Work out the finished part from the listing and answer in its coordinate system (mm). Give positions to 0.01 mm unless a question says otherwise; leave off trailing zeros. Loops run counter-clockwise (first coordinate to the right, second up) from the corner with the lowest first, then second, coordinate; pieces in that order, holes last. Notation, with made-up numbers: (54, 85) - (70, 85) arc R17 cw to (70, 104) - close; hole circle Ø1 at (0, 85.5). An arc over 180 degrees is marked (long way). One line per question, with ' | ' between items.
from build123d import *

# Parameters (mm, degrees)
SKETCH1_R           = 2.55
BOSS_EXTRUDE1_DEPTH = 3
FILLET1_R           = 2


with BuildPart() as part:
    # Sketch1 → Boss-Extrude1 (new body)
    with BuildSketch(Plane.XY):
        Polygon((-100, 96), (100, 96), (110, 96), (110, 4), (-110, 4), (-110, 96), align=None)
        with Locations((105, 20.245379956)):
            Circle(SKETCH1_R, mode=Mode.SUBTRACT)
        with Locations((105, 79.754620044)):
            Circle(SKETCH1_R, mode=Mode.SUBTRACT)
        with Locations((-105, 20.245379956)):
            Circle(SKETCH1_R, mode=Mode.SUBTRACT)
        with Locations((-105, 79.754620044)):
            Circle(SKETCH1_R, mode=Mode.SUBTRACT)
    extrude(amount=BOSS_EXTRUDE1_DEPTH)

    # Fillet1
    fillet1_edges = [part.edges().sort_by_distance(p)[0] for p in [
        (110, 4, 1.5),
        (-110, 4, 1.5),
        (-110, 96, 1.5),
        (110, 96, 1.5),
    ]]
    fillet(fillet1_edges, radius=FILLET1_R)


solid = part.part
1. Flat-ended cylindrical pins translate along their axes: pin 1 (6 mm diameter, centred on x = -36, y = 27.5, fed in from -Z); pin 2 (4 mm diameter, centred on x = -105, y = 79.75, fed in from -Z). Find the tip coordinate at first contact, or state that the pin passes through.
Evaluation:
pin 1: z = 0 | pin 2: through
2. Determine the mould class of faces 1 (the cylindrical face through (-102.568, 80.521, 1.479)), 2 (the cylindrical face through (107.432, 21.011, 1.479)), 3 (the flat face through (2, 51, 3)) for opening direction X: +X half, -X half, draft (parallel to the pull), parting line (faces both ways), or undercut.
Evaluation:
face 1: undercut | face 2: undercut | face 3: draft
3. Find section A-A on x = -105. Write down the section's boundary in (y, z).
Evaluation:
outline: (4, 0) - (17.7, 0) - (17.7, 3) - (4, 3) - close; (22.8, 0) - (77.2, 0) - (77.2, 3) - (22.8, 3) - close; (82.3, 0) - (96, 0) - (96, 3) - (82.3, 3) - close
4. Consider L1, parallel to Y at x = 105, z = 1.45. Determine where the line is inside the solid, lowest interval first.
Evaluation:
L1: 4 to 17.7, 22.8 to 77.2, 82.3 to 96
